```python
from build123d import *

# Parameters (mm, degrees)
BOSS_EXTRUDE3_DEPTH = 10
FILLET3_R           = 3


with BuildPart() as part:
    # Sketch1 → Boss-Extrude3 (new body)
    with BuildSketch(Plane(origin=(0, 0, 0), x_dir=(1, 0, 0), z_dir=(0, 1, 0))):
        with BuildLine():
            Line((-56.127249733, 13.064532605), (-51.956028901, 16.165106996))
            ThreePointArc((-51.956028901, 16.165106996), (-63.652726326, 23.094481669), (-76.795589263, 19.616821846))
            ThreePointArc((-76.795589263, 19.616821846), (-77.629630472, 18.791218581), (-78.553962744, 18.068131215))
            ThreePointArc((-78.553962744, 18.068131215), (-79.603636657, 16.913208133), (-80.546816269, 15.669795544))
            ThreePointArc((-80.546816269, 15.669795544), (-94.691323687, 5.670927287), (-80.546816269, -4.32794097))
            ThreePointArc((-80.546816269, -4.32794097), (-79.603636657, -5.571353559), (-78.553962744, -6.726276641))
            ThreePointArc((-78.553962744, -6.726276641), (-77.629630472, -7.449364007), (-76.795589263, -8.274967272))
            ThreePointArc((-76.795589263, -8.274967272), (-63.652726326, -11.752627095), (-51.956028901, -4.823252422))
            Line((-51.956028901, -4.823252422), (-56.127249733, -1.722678031))
            ThreePointArc((-56.127249733, -1.722678031), (-66.96819929, -6.690371176), (-76.981216312, -0.213979234))
            ThreePointArc((-76.981216312, -0.213979234), (-79.478589631, 0.394605678), (-82.048720515, 0.435548601))
            ThreePointArc((-82.048720515, 0.435548601), (-89.702342556, 5.670927287), (-82.048720515, 10.906305973))
            ThreePointArc((-82.048720515, 10.906305973), (-79.478589631, 10.947248896), (-76.981216312, 11.555833808))
            ThreePointArc((-76.981216312, 11.555833808), (-66.96819929, 18.03222575), (-56.127249733, 13.064532605))
        make_face()
    extrude(amount=BOSS_EXTRUDE3_DEPTH)

    # Fillet3
    fillet3_edges = [part.edges().sort_by_distance(p)[0] for p in [
        (-51.956028901, 5, 4.823252422),
        (-80.546816269, 5, 4.32794097),
        (-80.546816269, 5, -15.669795544),
        (-51.956028901, 5, -16.165106996),
    ]]
    fillet(fillet3_edges, radius=FILLET3_R)


solid = part.part
```
Verification items for the finished model (mm, model axes). A direction names the side the tool comes from. Round coordinates to 2 decimals unless told otherwise and drop trailing zeros. Order: outer loops, then holes, each group sorted by start corner. A loop starts at its lowest first (then second) coordinate and runs counter-clockwise, first axis right, second up. Notation, with made-up numbers: (85, 2) -> (113, 2) arc R16 cw to (113, 9) -> close; hole circle Ø1 at (-29.75, 12). An arc over 180 degrees is marked (long way). Put each result on its own line as item: value. Start each with the question number.
(1) Material ranges on line 1 along Z through (x, y) = (-84, 0.75); line 2 along X through (y, z) = (6.75, 3); line 3 along Z through (x, y) = (-72, 6), recorded low to high.
(2) Section check B-B (x = -77.5). Enter the section's corners in (y, z).
(3) Section check C-C (z = -3.5). Enter the section's corners in (x, y), then the cut area to 3 significant figures.
(4) Tool access check on faces 5 (the face through (-66.8, 4.9, 6.7)), 6 (the face through (-55.38, 4.93, -13.62)), 7 (the face through (-76, 10, -14)). Record the directions out of +Z, -Z, +X, -X, +Y, -Y that give a thin tool (end or side, any length) a straight path to the whole face; none if there is none.
(5) Depth check by flat-ended pin: pin 1 Ø6 at (y, z) = (3.5, 0) entering from -X; pin 2 Ø2 at (x, y) = (-81.5, 1.5) entering from -Z; pin 3 Ø1 at (y, z) = (8.5, -2) entering from -X. Enter the tip coordinate at first touch or a pass-through.
(6) Section check D-D (x = -90.5). Enter the section's corners in (y, z), then the cut area to 3 significant figures.
(7) Draft check along Z on faces 1 (the face through (-53.41, 5.07, -16.43)), 2 (the face through (-79.01, 4.93, 6.25)), 3 (the face through (-94.69, 4.93, -5.93)), 4 (the face through (-65.297, 4.93, -23.245)). Enter one of: +Z half, -Z half, draft (parallel to the pull), parting line (faces both ways), or undercut.
(8) Section check A-A (x = -67.5). Enter the section's corners in (y, z).
Completed:
1. line 1: z = -16.28 to -11.29, -0.05 to 4.94
1. line 2: x = -90.19 to -74.93, -57.22 to -54.43
1. line 3: z = -22.23 to -16.56, 5.21 to 10.89
2. outline: (0, -18.91) -> (10, -18.91) -> (10, -11.38) -> (0, -11.38) -> close; (0, 0.04) -> (10, 0.04) -> (10, 7.57) -> (0, 7.57) -> close
3. outline: (-94.47, 0) -> (-89.27, 0) -> (-89.27, 10) -> (-94.47, 10) -> close
3. area: 52.0 mm2
4. face 5: +Y, -Y
4. face 6: +X, +Y, -Y
4. face 7: +Z, -Z, +X, -X, +Y
5. pin 1: stops at x = -94.35
5. pin 2: stops at z = -16.32
5. pin 3: stops at x = -94.21
6. outline: (0, -14.12) -> (10, -14.12) -> (10, 2.78) -> (0, 2.78) -> close
6. area: 169 mm2
7. face 1: undercut
7. face 2: +Z half
7. face 3: parting line
7. face 4: -Z half
8. outline: (0, -23.2) -> (10, -23.2) -> (10, -17.98) -> (0, -17.98) -> close; (0, 6.64) -> (10, 6.64) -> (10, 11.86) -> (0, 11.86) -> close
